Source: CAD feature listing. Evaluate the final solid. Frame: model axes, mm. A direction names the side the tool comes from. Round coordinates to 2 decimals unless told otherwise and drop trailing zeros. Order: outer loops, then holes, each group sorted by start corner. A loop starts at its lowest first (then second) coordinate and runs counter-clockwise, first axis right, second up. Notation, with made-up numbers: (-16.75, 20.5) - (-7.75, 20.5) arc R27 ccw to (-7.75, 57.5) - close; hole circle Ø1 at (58.25, 60). An arc over 180 degrees is marked (long way). Return JSON: item names as keys, results as strings. Group by question number.
1) Section D-D, the plane y = 8. Return loops of the section in (x, z), plus the area to 3 significant figures.
2) Contact query for flat-ended pins moving along their axis: P1, Ø8, axis at y = 15.5, z = 60, coming from the -X side; P2, Ø6, axis at y = 6.5, z = 43, coming from the +X side (3 decimals); P3, Ø1, axis at y = 15, z = 39, coming from the -X side. Output: stop coordinate, or through.
3) Access query for faces 5 (the flat face through (-19.5, 9, 63)), 6 (the cylindrical face through (0, 0, 63)), 7 (the flat face through (8, 2, 43)). Directions: +Z, -Z, +X, -X, +Y, -Y. A direction counts if a zero-diameter tool reaches every point of the face in a straight line with its end or side. Return the directions, or none.
4) Ray query, line 1 (X direction, y = 3.75, z = -8); line 2 (X direction, y = 12, z = 68); line 3 (Y direction, x = -18.5, z = 15). Return the intervals inside material, ascending. Write a range as from..to.
5) Section A-A, the plane z = 75.5. Return loops of the section in (x, y), plus the area to 3 significant figures.
6) Section C-C, the plane x = -4.5. Return loops of the section in (y, z), plus the area to 3 significant figures.
7) Section B-B, the plane y = 3.5. Return loops of the section in (x, z).
8) Mould query, pull axis Z, two halves, no side actions, for faces 1 (the flat face through (0, -1, 83)), 2 (the flat face through (-23, 9, 0)), 3 (the flat face through (-19.826, 10.14, 21)), 4 (the flat face through (0, 9, -23)). Classes: pulls with the +Z half, pulls with the -Z half, needs draft (parallel to the pull), parting line crosses it, or undercut.
```python
from build123d import *

# Parameters (mm, degrees)
SKETCH1_W           = 46
SKETCH1_H           = 46
SKETCH1_W_2         = 40
SKETCH1_H_2         = 40
BOSS_EXTRUDE1_DEPTH = 20
SKETCH2_W           = 46
SKETCH2_H           = 46
BOSS_EXTRUDE2_DEPTH = 2
BOSS_EXTRUDE3_DEPTH = 22
CUT_EXTRUDE1_DEPTH  = 20
BOSS_EXTRUDE5_DEPTH = 2
BOSS_EXTRUDE6_DEPTH = 40
BOSS_EXTRUDE8_DEPTH = 20
SKETCH12_R          = 2.55
CUT_EXTRUDE4_DEPTH  = 20


with BuildPart() as part:
    # Sketch1 → Boss-Extrude1 (new body)
    with BuildSketch(Plane(origin=(0, 0, 0), x_dir=(1, 0, 0), z_dir=(0, 1, 0))):
        Rectangle(SKETCH1_W, SKETCH1_H)
        Rectangle(SKETCH1_W_2, SKETCH1_H_2, mode=Mode.SUBTRACT)
    extrude(amount=BOSS_EXTRUDE1_DEPTH)

    # Sketch2 → Boss-Extrude2 (add)
    with BuildSketch(Plane.XZ):
        Rectangle(SKETCH2_W, SKETCH2_H)
    extrude(amount=BOSS_EXTRUDE2_DEPTH)

    # Sketch3 → Boss-Extrude3 (add)
    with BuildSketch(Plane(origin=(0, 20, 0), x_dir=(1, 0, 0), z_dir=(0, 1, 0))):
        Polygon((-16, -43), (-19.47826087, -23), (-23, -23), (-19.5, -43), align=None)
        Polygon((23, -23), (19.47826087, -23), (16, -43), (19.5, -43), align=None)
    extrude(amount=-BOSS_EXTRUDE3_DEPTH)

    # Sketch3<3> → Cut-Extrude1 (cut)
    with BuildSketch(Plane(origin=(0, 20, 0), x_dir=(1, 0, 0), z_dir=(0, 1, 0))):
        Polygon((20, -20), (-20, -20), (-19.47826087, -23), (19.47826087, -23), align=None)
    extrude(amount=-CUT_EXTRUDE1_DEPTH, mode=Mode.SUBTRACT)

    # Sketch5 → Boss-Extrude5 (add)
    with BuildSketch(Plane.XZ.offset(2)):
        Polygon((-16, 43), (-19.47826087, 23), (19.47826087, 23), (16, 43), align=None)
    extrude(amount=-BOSS_EXTRUDE5_DEPTH)

    # Sketch6 → Boss-Extrude6 (add)
    with BuildSketch(Plane.XY.offset(43)):
        with BuildLine():
            Line((-10, 10), (-10, 20))
            Line((-10, 20), (-19.5, 20))
            Line((-19.5, 20), (-19.5, -2))
            Line((-19.5, -2), (19.5, -2))
            Line((19.5, -2), (19.5, 20))
            Line((19.5, 20), (10, 20))
            Line((10, 20), (10, 10))
            ThreePointArc((10, 10), (0, 0), (-10, 10))
        make_face()
    extrude(amount=BOSS_EXTRUDE6_DEPTH)

    # Sketch10 → Boss-Extrude8 (add)
    with BuildSketch(Plane(origin=(0, 20, 0), x_dir=(1, 0, 0), z_dir=(0, 1, 0))):
        with BuildLine():
            ThreePointArc((-10, -43), (-16.076894226, -33.091178776), (-19.647093187, -22.029214175))
            Line((-19.647093187, -22.029214175), (-16, -43))
            Line((-16, -43), (-10, -43))
        make_face()
        with BuildLine():
            Line((16, -43), (20, -20))
            ThreePointArc((20, -20), (16.354828561, -32.089055896), (10, -43))
            Line((10, -43), (16, -43))
        make_face()
    extrude(amount=-BOSS_EXTRUDE8_DEPTH)

    # Sketch12 → Cut-Extrude4 (cut)
    with BuildSketch(Plane(origin=(-26.221952699, 0, 4.588841722), x_dir=(0.17238033175224893, 0, 0.9850304671557041), z_dir=(-0.9850304671557042, 0, 0.17238033175224893))):
        with Locations((25.097340794, 15.70534694)):
            Circle(SKETCH12_R)
    extrude(amount=-CUT_EXTRUDE4_DEPTH, mode=Mode.SUBTRACT)


solid = part.part
```
Geometry check:
{
 "1": {"outline": "(-23, -23) - (23, -23) - (23, 23) - (19.5, 43) - (19.5, 83) - (9.8, 83) - (9.8, 43) - (10, 43) arc R53.96 cw to (20, 20) - (20, -20) - (-20, -20) - (-20, 20) - (-19.65, 22.03) arc R48.97 cw to (-10, 43) - (-9.8, 43) - (-9.8, 83) - (-19.5, 83) - (-19.5, 43) - (-23, 23) - close", "area": "1,400 mm2"},
 "2": {"P1": "x = -19.5", "P2": "x = 20.025", "P3": "x = -20.29"},
 "3": {"face 5": "+Z, -X, +Y, -Y", "face 6": "+Z, +Y", "face 7": "+Y"},
 "4": {"line 1": "-23..-20, 20..23", "line 2": "-19.5..-10, 10..19.5", "line 3": "-2..0"},
 "5": {"outline": "(-19.5, -2) - (19.5, -2) - (19.5, 20) - (10, 20) - (10, 10) arc R10 cw to (-10, 10) - (-10, 20) - (-19.5, 20) - close", "area": "501 mm2"},
 "6": {"outline": "(-2, -23) - (20, -23) - (20, -20) - (0, -20) - (0, 43) - (1.07, 43) - (1.07, 83) - (-2, 83) - close", "area": "315 mm2"},
 "7": {"outline": "(-23, -23) - (23, -23) - (23, 23) - (19.5, 43) - (19.5, 83) - (7.6, 83) - (7.6, 43) - (10, 43) arc R53.96 cw to (20, 20) - (20, -20) - (-20, -20) - (-20, 20) - (-19.65, 22.03) arc R48.97 cw to (-10, 43) - (-7.6, 43) - (-7.6, 83) - (-19.5, 83) - (-19.5, 43) - (-23, 23) - close"},
 "8": {"face 1": "pulls with the +Z half", "face 2": "needs draft", "face 3": "undercut", "face 4": "pulls with the -Z half"}
}
